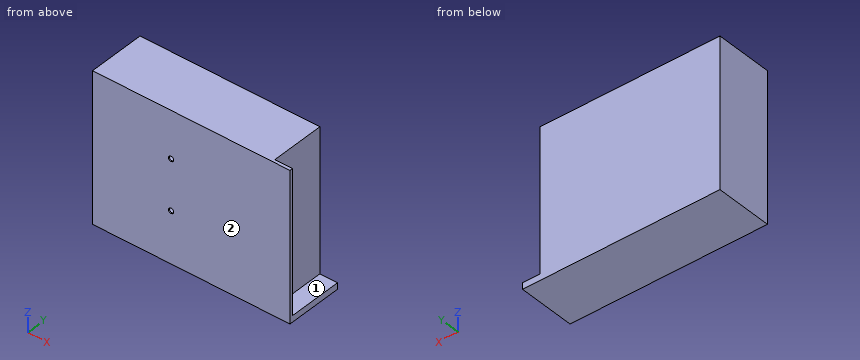
from build123d import *

# Parameters (mm, degrees)
SKETCH1_W                = 129.5
SKETCH1_H                = 97.5
BOSS_EXTRUDE1_DEPTH      = 37.5
M3_CLEARANCE_HOLE1_D     = 3.4
M3_CLEARANCE_HOLE1_DEPTH = 0.737
M3_CLEARANCE_HOLE1_TIP   = 1.021463052
SKETCH5_W                = 11.575237046
SKETCH5_H                = 93.370280938
CUT_EXTRUDE1_DEPTH       = 35.5


with BuildPart() as part:
    # Sketch1 → Boss-Extrude1 (new body)
    with BuildSketch(Plane(origin=(0, 0, 0), x_dir=(1, 0, 0), z_dir=(0, 1, 0))):
        with Locations((64.75, 48.75)):
            Rectangle(SKETCH1_W, SKETCH1_H)
    extrude(amount=BOSS_EXTRUDE1_DEPTH)

    # M3 Clearance Hole1
    with Locations(Plane(origin=(0, 0, 0), x_dir=(-1, 0, 0), z_dir=(0, -1, 0))):
        with Locations((-51.5, 63.75), (-51.5, 30.75)):
            Hole(M3_CLEARANCE_HOLE1_D / 2, depth=M3_CLEARANCE_HOLE1_DEPTH)
            with Locations((0, 0, -(M3_CLEARANCE_HOLE1_DEPTH + M3_CLEARANCE_HOLE1_TIP / 2))):  # 118° drill point
                Cone(0, M3_CLEARANCE_HOLE1_D / 2, M3_CLEARANCE_HOLE1_TIP, mode=Mode.SUBTRACT)

    # Sketch5 → Cut-Extrude1 (cut)
    with BuildSketch(Plane(origin=(0, 37.5, 0), x_dir=(1, 0, 0), z_dir=(0, 1, 0))):
        with Locations((123.712381477, 46.685140469)):
            Rectangle(SKETCH5_W, SKETCH5_H)
    extrude(amount=-CUT_EXTRUDE1_DEPTH, mode=Mode.SUBTRACT)


solid = part.part
Model file for the job. Use its own axes, mm. Face numbers are marked on the shaded views. A direction names the side the tool comes from. Round coordinates to 2 decimals unless told otherwise and drop trailing zeros. Loops run counter-clockwise (first coordinate to the right, second up) from the corner with the lowest first, then second, coordinate; pieces in that order, holes last. Notation, with made-up numbers: (70.5, 7) - (94.5, 7) arc R29 ccw to (94.5, 31) - close; hole circle Ø11 at (64, -6). An arc over 180 degrees is marked (long way). Write each question's results on one line, items separated by ' | '.
(1) Pin check, flat tips, straight feed: pin 1 (6 mm diameter, centred on x = 125, z = -66, fed in from +Y); pin 2 (9.5 mm diameter, centred on x = 125, y = 17, fed in from +Z); pin 3 (4 mm diameter, centred on y = 16, z = -79, fed in from +X). Stop position of each tip, or through.
Answer below:
pin 1: stops at y = 2 | pin 2: stops at z = -93.37 | pin 3: stops at x = 117.92
(2) Wall check: L1, parallel to X at y = 0.15, z = -30.75; L2, parallel to X at y = 23, z = -81.5; L3, parallel to Z at x = 118, y = 8. Give the ranges that are in metal, low to high.
Answer below:
L1: x = 0 to 49.8, 53.2 to 129.5 | L2: x = 0 to 117.92 | L3: z = -97.5 to -93.37
(3) Saw through at A-A, the plane y = 5. List the corners of the cut face in (x, z).
Answer below:
outline: (0, -97.5) - (129.5, -97.5) - (129.5, -93.37) - (117.92, -93.37) - (117.92, 0) - (0, 0) - close
(4) 3-axis set-ups, long thin cutter, end or side, ignore diameter. For the marked faces 1 and 2: which of +Z, -Z, +X, -X, +Y, -Y reach the whole face in a straight line?
Answer below:
face 1: +Z, +X, +Y | face 2: +Z, -Z, +X, -X, -Y
